from build123d import *

# Parameters (mm, degrees)
F1_DEPTH  = 50
F3_W      = 220
F3_H      = 40
F4_DEPTH  = 760
F5_DEPTH  = 240
F6_W      = 319.9999928474
F6_H      = 220
F6_W_2    = 280
F6_H_2    = 180
F7_DEPTH  = 50
F8_DEPTH  = 435.9292732552
F9_W      = 140
F9_H      = 220
F10_DEPTH = 10
F12_DEPTH = 240
F13_DEPTH = 25
F14_DEPTH = 25
F16_W     = 220
F16_H     = 40
F17_DEPTH = 5
F15_W     = 220
F15_H     = 40
F18_DEPTH = 5


with BuildPart() as f1:
    # F0 (on Top) → F1 (new body)
    with BuildSketch(Plane.XY):
        Polygon((-178.3412894642, 148.3412835037), (-380, 120), (-380, -120), (-178.3412894642, -148.3412835037), (-150.0000059605, -120), (150.0000059605, -120), (178.3412894642, -148.3412835037), (380, -120), (380, 120), (178.3412894642, 148.3412835037), (150.0000059605, 120), (-150.0000059605, 120), align=None)
    extrude(amount=F1_DEPTH)

    # F3 (on face) → F4 (cut)
    with BuildSketch(Plane(origin=(-380, 0, 0), x_dir=(0, -1, 0), z_dir=(-1, 0, 0))):
        with Locations((0, 25)):
            Rectangle(F3_W, F3_H)
    extrude(amount=-F4_DEPTH, mode=Mode.SUBTRACT)

    # F2 (on face) → F5 (cut)
    with BuildSketch(Plane.XZ.offset(120)):
        Polygon((305, 0), (380, 0), (380, 35), (340, 35), align=None)
        Polygon((-340, 35), (-380, 35), (-380, 0), (-305, 0), align=None)
    extrude(amount=-F5_DEPTH, mode=Mode.SUBTRACT)

    # F6 (on face) → F7 (cut)
    with BuildSketch(Plane.XY.offset(50)):
        Rectangle(F6_W, F6_H)
        Rectangle(F6_W_2, F6_H_2, mode=Mode.SUBTRACT)
    extrude(amount=-F7_DEPTH, mode=Mode.SUBTRACT)

    # F2 (on face) → F8 (cut, symmetric)
    with BuildSketch(Plane.XZ.offset(120)):
        Polygon((-340, 35), (-380, 35), (-380, 0), (-305, 0), align=None)
        Polygon((305, 0), (380, 0), (380, 35), (340, 35), align=None)
    extrude(amount=F8_DEPTH, both=True, mode=Mode.SUBTRACT)

    # F9 (on face) → F10 (cut)
    with BuildSketch(Plane.XY.offset(50)):
        with Locations((-234.9999964237, 0)):
            Rectangle(F9_W, F9_H)
        with Locations((234.9999964237, 0)):
            Rectangle(F9_W, F9_H)
    extrude(amount=-F10_DEPTH, mode=Mode.SUBTRACT)

    # F11 (on face) → F12 (join)
    with BuildSketch(Plane.XZ.offset(120)):
        Polygon((-305.0000059605, 0), (-305.0000059605, 7.0710678119), (-332.9289381486, 35), (-340.0000059605, 35), align=None)
        Polygon((340.0000059605, 35), (332.9289381486, 35), (305.0000059605, 7.0710678119), (305.0000059605, 0), align=None)
    extrude(amount=-F12_DEPTH)

    # F13 (cut): a face of the model
    f13_faces = [f1.faces().sort_by_distance(p)[0] for p in [
        (0, 0, 50),
    ]]
    extrude(f13_faces, amount=-F13_DEPTH, mode=Mode.SUBTRACT)

    # F14 (cut): a face of the model
    f14_faces = [f1.faces().sort_by_distance(p)[0] for p in [
        (0, 0, 0),
    ]]
    extrude(f14_faces, amount=-F14_DEPTH, mode=Mode.SUBTRACT)

    # F16 (on face) → F17 (join)
    with BuildSketch(Plane.YZ.offset(-159.9999964237)):
        with Locations((0, 25)):
            Rectangle(F16_W, F16_H)
    extrude(amount=-F17_DEPTH)

    # F15 (on face) → F18 (join)
    with BuildSketch(Plane(origin=(159.9999964237, 0, 0), x_dir=(0, -1, 0), z_dir=(-1, 0, 0))):
        with Locations((0, 25)):
            Rectangle(F15_W, F15_H)
    extrude(amount=-F18_DEPTH)


solid = f1.part
Could you check a few things on this model? Use its own coordinates, in mm. A direction names the side the tool comes from. Round coordinates to 2 decimals unless told otherwise and drop trailing zeros. Write each loop counter-clockwise with the first axis right and the second up, starting at its lowest first coordinate (ties: lowest second). Pieces come first, ordered by that corner, then holes. Notation, with made-up numbers: (40, -2) - (67, -2) arc R14 cw to (67, 3) - close; hole circle Ø10 at (73, -34.75). An arc over 180 degrees is marked (long way). Put each result on its own line as item: value. Start each with the question number.
(1) Will these pins go through, and if not, where does the flat tip stop? pin 1 (3 mm diameter, centred on x = 74.5, z = 9, fed in from -Y); pin 2 (1.5 mm diameter, centred on y = 53.5, z = 17.5, fed in from +X); pin 3 (1.5 mm diameter, centred on y = 53, z = 7, fed in from -X).
(2) I want a section at B-B, the plane y = 28.5. Give the number of separate pieces and of enclosed holes in the cut face, plus the area to 3 significant figures.
(3) I need wall thicknesses on probe 1 along X at (y, z) = (-10, 45.5); probe 2 along X at (y, z) = (6.5, 8); probe 3 along Y at (x, z) = (-10, 36.5). Which ranges of each line are inside material? Lowest first, please.
(4) For faces 4 (the flat face through (342, 2, 45)), 5 (the flat face through (319.16, -1.54, 21.23)), 6 (the flat face through (-164, 134, 25)), 7 (the flat face through (-2, -120, 25)), 8 (the flat face through (-160, -2, 25)), which set-ups out of +Z, -Z, +X, -X, +Y, -Y let a thin tool reach every point of the face, with its end or its side?
(5) I want a section at A-A, the plane x = 25.5. Please give me the cut outline in (y, z), plus the area to 3 significant figures.
(6) Thinking about a two-plate mould opening in Y: for faces 1 (the flat face through (2, 120, 25)), 2 (the flat face through (234, 2, 5)), 3 (the flat face through (360, -116, 35)), which applies, released by +Y, released by -Y, zero draft, split by the parting line, or undercut?
(7) I want a section at D-D, the plane x = 245. Please give me the cut outline in (y, z).
Here are the results:
1. pin 1: stops at y = -120
1. pin 2: stops at x = 323.25
1. pin 3: stops at x = -312.75
2. separate pieces: 4
2. enclosed holes: 0
2. area: 3,090 mm^2
3. probe 1: x = -380 to -305, -165 to -160, 160 to 165, 305 to 380
3. probe 2: x = -313 to -305.93, -165 to -160, 160 to 165, 305.93 to 313
3. probe 3: y = -120 to -110, 110 to 120
4. face 4: +X
4. face 5: none
4. face 6: +Z, -Z, +Y
4. face 7: +Z, -Z, -Y
4. face 8: +Z, -Z
5. outline: (-120, 0) - (-110, 0) - (-110, 50) - (-120, 50) - close; (110, 0) - (120, 0) - (120, 50) - (110, 50) - close
5. area: 1,000 mm^2
6. face 1: released by +Y
6. face 2: undercut
6. face 3: zero draft
7. outline: (-138.97, 0) - (138.97, 0) - (138.97, 50) - (110, 50) - (110, 5) - (-110, 5) - (-110, 50) - (-138.97, 50) - close
